Geometry: final body of the model. Coordinates: model frame, mm. A direction names the side the tool comes from. Give positions to 0.01 mm unless a question says otherwise; leave off trailing zeros. Order: outer loops, then holes, each group sorted by start corner. A loop starts at its lowest first (then second) coordinate and runs counter-clockwise, first axis right, second up. Notation, with made-up numbers: (71, -38) -> (115, -38) arc R28 cw to (115, 1) -> close; hole circle Ø11 at (54.5, 34). An arc over 180 degrees is marked (long way). Answer in a Markdown table with one row per item. Add a question column.
Q1. Contact query for flat-ended pins moving along their axis: P1, Ø3.5, axis at x = -8, z = 3, coming from the -Y side; P2, Ø10, axis at x = -12.5, y = 14, coming from the -Z side; P3, Ø4.5, axis at y = 14.5, z = 4, coming from the -X side. Output: stop coordinate, or through.
Q2. Pull-direction query (Y, two-part tool) for faces 1 (the face through (2, -6, -2)), 2 (the face through (-19, 10, 3)), 3 (the face through (-2, 1.1, 5)); classes: +Y half, -Y half, draft (parallel to the pull), parting line (faces both ways), or undercut.
Q3. Cut plane B-B on y = 13.75. Return the cut outline in (x, z).
Q4. Cut plane D-D on z = 3. Return the cut outline in (x, y) (3 decimals), and give its area (3 significant figures).
Q5. Line query: line 1 along Y through (x, z) = (-6.5, 3); line 2 along Y through (x, z) = (5, 9.5) (3 decimals); line 3 along Y through (x, z) = (10.5, 3.5). Output: solid intervals per line, ascending. Write a range as from..to.
Q6. Set-up query: faces 4 (the face through (13, 4.2, 7.9)), 5 (the face through (-15, 2, 9)), 6 (the face through (1, 12, 6.85)). Return all of +Z, -Z, +X, -X, +Y, -Y with unobstructed straight access to the full face (end or side cutting, diameter ignored); none if empty.
Q7. Cut plane A-A on z = 5.25. Return the cut outline in (x, y) (3 decimals), and give its area (3 significant figures).
Q8. Cut plane C-C on x = 11.5. Return the cut outline in (y, z).
from build123d import *

# Parameters (mm, degrees)
BOSS_EXTRUDE1_DEPTH     = 20
BOSS_EXTRUDE4_DEPTH     = 6
CHAMFER4_SIZE           = 5
BOSS_EXTRUDE5_DEPTH     = 4
CUT_EXTRUDE4_DEPTH      = 33.573148451
CUT_EXTRUDE4_DEPTH_BACK = 33.573148451
FILLET1_R               = 10
CHAMFER5_SIZE           = 2.5
SKETCH17_W              = 9
SKETCH17_H              = 1.25
CUT_EXTRUDE5_DEPTH      = 33.573148451
SKETCH18_W              = 8
SKETCH18_H              = 9.375
BOSS_EXTRUDE6_DEPTH     = 4
BOSS_EXTRUDE8_REACH     = 33.067


with BuildPart() as part:
    # Sketch1 → Boss-Extrude1 (new, symmetric)
    with BuildSketch(Plane(origin=(0, 0, 0), x_dir=(0, 0, -1), z_dir=(1, 0, 0))):
        Polygon((0, -6), (4, -6), (-0.849880383, 12.1), (-6.849880383, 12.1), (-6.849880383, 5.250119617), (-9, 3.1), (-9, 1.1), (0, 1.1), (0, 0), (-8.56888804, 0), align=None)
    extrude(amount=BOSS_EXTRUDE1_DEPTH, both=True)

    # Sketch7 → Boss-Extrude4 (add)
    with BuildSketch(Plane.XY.offset(6.849880383)):
        with BuildLine():
            Line((-20, 12.1), (-20, 20.1))
            Line((-20, 20.1), (-16.941074346, 20.1))
            ThreePointArc((-16.941074346, 20.1), (0, 13.1), (16.941074346, 20.1))
            Line((16.941074346, 20.1), (20, 20.1))
            Line((20, 20.1), (20, 12.1))
            Line((20, 12.1), (-20, 12.1))
        make_face()
    extrude(amount=-BOSS_EXTRUDE4_DEPTH)

    # Chamfer4
    chamfer4_edges = [part.edges().sort_by_distance(p)[0] for p in [
        (-18.470537173, 20.1, 6.849880383),
        (18.470537173, 20.1, 6.849880383),
    ]]
    chamfer(chamfer4_edges, length=CHAMFER4_SIZE)

    # Sketch15 → Boss-Extrude5 (add)
    with BuildSketch(Plane.ZY.offset(20)):
        Polygon((9, 1.1), (9, 3.1), (6.849880383, 5.250119617), (6.849880383, 15.1), (1.849880383, 20.1), (0.849880383, 20.1), (0.849880383, 12.1), (-4, -6), (0, -6), (8.56888804, 0), (0, 0), (0, 1.1), align=None)
    extrude(amount=BOSS_EXTRUDE5_DEPTH)

    # Sketch16 → Cut-Extrude4 (cut, two sides: drawn at the far end of the back side and taken through both)
    with BuildSketch(Plane.XY.offset(-CUT_EXTRUDE4_DEPTH_BACK)):
        Polygon((-24, 1.1), (-19, 3.986751346), (-19, 20.1), (-24, 20.1), align=None)
    extrude(amount=CUT_EXTRUDE4_DEPTH + CUT_EXTRUDE4_DEPTH_BACK, mode=Mode.SUBTRACT)

    # Fillet1
    # the kernel refuses this fillet: 10 mm, written as the material it takes off along each edge
    with BuildSketch(Plane(origin=(-24, -6, -27.925666135), x_dir=(1, 0, 0), z_dir=(0, 0, 1))) as fillet1_piece_1:
        with BuildLine():
            CenterArc((9.570266454, 10), FILLET1_R, 196.857956022, 73.142043978)
            Line((0, 7.1), (-0.191405329, 7.042))
            ThreePointArc((-0.191405329, 7.042), (-0.2, 3.55), (-0.2, 0))
            Line((-0.2, 0), (0, -0.2))
            Line((0, -0.2), (9.570266454, -0.2))
            Line((9.570266454, -0.2), (9.570266454, 0))
        make_face()
    extrude(amount=51.85133227, mode=Mode.SUBTRACT)

    # Chamfer5
    chamfer5_edges = [part.edges().sort_by_distance(p)[0] for p in [
        (20, -6, -2),
    ]]
    chamfer(chamfer5_edges, length=CHAMFER5_SIZE)

    # Sketch17 → Cut-Extrude5 (cut, through all)
    with BuildSketch(Plane.XY):
        with Locations((0, 11.1)):
            Rectangle(SKETCH17_W, SKETCH17_H)
    extrude(amount=CUT_EXTRUDE5_DEPTH, mode=Mode.SUBTRACT)

    # Sketch18 → Boss-Extrude6 (add)
    with BuildSketch(Plane.XY.offset(6.849880383)):
        with Locations((0, 5.7875)):
            Rectangle(SKETCH18_W, SKETCH18_H)
    extrude(amount=BOSS_EXTRUDE6_DEPTH)

    # Boss-Extrude8: up to this face of the body (flat: up to its plane)
    boss_extrude8_end = Plane(part.part.faces().sort_by_distance((-1.927949963, 1.1, 4.69543357))[0])
    # Sketch19 → Boss-Extrude8 (add, up to the picked face)
    with BuildSketch(Plane(origin=(0, 10.475, 0), x_dir=(1, 0, 0), z_dir=(0, 1, 0)), mode=Mode.PRIVATE) as boss_extrude8_sk1:
        Polygon((4, -6.849880383), (4, -10.849880383), (8, -6.849880383), align=None)
    boss_extrude8_tool1 = split(extrude(boss_extrude8_sk1.sketch, amount=-BOSS_EXTRUDE8_REACH, mode=Mode.PRIVATE), bisect_by=boss_extrude8_end, keep=Keep.BOTH, mode=Mode.PRIVATE)
    # Sketch19 → Boss-Extrude8 (add, up to the picked face)
    with BuildSketch(Plane(origin=(0, 10.475, 0), x_dir=(1, 0, 0), z_dir=(0, 1, 0)), mode=Mode.PRIVATE) as boss_extrude8_sk2:
        Polygon((-4, -6.849880383), (-8, -6.849880383), (-4, -10.849880383), align=None)
    boss_extrude8_tool2 = split(extrude(boss_extrude8_sk2.sketch, amount=-BOSS_EXTRUDE8_REACH, mode=Mode.PRIVATE), bisect_by=boss_extrude8_end, keep=Keep.BOTH, mode=Mode.PRIVATE)
    add(boss_extrude8_tool1.solids().sort_by(Axis((5.333333, 10.475, 8.183214), (0, -1, 0)))[0])
    add(boss_extrude8_tool2.solids().sort_by(Axis((-5.333333, 10.475, 8.183214), (0, -1, 0)))[0])


solid = part.part
Completed:
| question | item | result |
|---|---|---|
| 1 | P1 | stops at y = -5.12 |
| 1 | P2 | stops at z = 0.02 |
| 1 | P3 | stops at x = -19 |
| 2 | face 1 | -Y half |
| 2 | face 2 | draft |
| 2 | face 3 | undercut |
| 3 | outline | (-19, 0.85) -> (-5.55, 0.85) -> (-5.55, 6.85) -> (-19, 6.85) -> close; (5.55, 0.85) -> (20, 0.85) -> (20, 6.85) -> (5.55, 6.85) -> close |
| 4 | outline | (-24, 1.1) -> (20, 1.1) -> (20, 18.95) -> (15.703, 18.95) arc R24 cw to (-15.703, 18.95) -> (-19, 18.95) -> (-19, 3.987) -> close; (-23.595, 0) arc R10 ccw to (-20.562, -3.899) -> (19.601, -3.899) -> (20, -3.5) -> (20, 0) -> close; hole (-4.5, 10.475) -> (4.5, 10.475) -> (4.5, 11.725) -> (-4.5, 11.725) -> close |
| 4 | area | 731 mm² |
| 5 | line 1 | y = -3.9..0, 1.1..14 |
| 5 | line 2 | y = 1.1..10.475 |
| 5 | line 3 | y = -3.55..0, 1.1..15.52 |
| 6 | face 4 | +Z, +X, +Y |
| 6 | face 5 | +Z, -X, +Y, -Y |
| 6 | face 6 | +Z, +Y |
| 7 | outline | (-24, 1.1) -> (20, 1.1) -> (20, 16.7) -> (12.643, 16.7) arc R24 cw to (-12.643, 16.7) -> (-19, 16.7) -> (-19, 3.987) -> close; (-23.595, 0) arc R10 ccw to (-22.176, -2.324) -> (20, -2.324) -> (20, 0) -> close; hole (-4.5, 10.475) -> (4.5, 10.475) -> (4.5, 11.725) -> (-4.5, 11.725) -> close |
| 7 | area | 643 mm² |
| 8 | outline | (-6, -4) -> (12.1, 0.85) -> (16.03, 0.85) -> (16.03, 5.92) -> (15.1, 6.85) -> (5.25, 6.85) -> (3.1, 9) -> (1.1, 9) -> (1.1, 0) -> (0, 0) -> (0, 8.57) -> (-6, 0) -> close |
